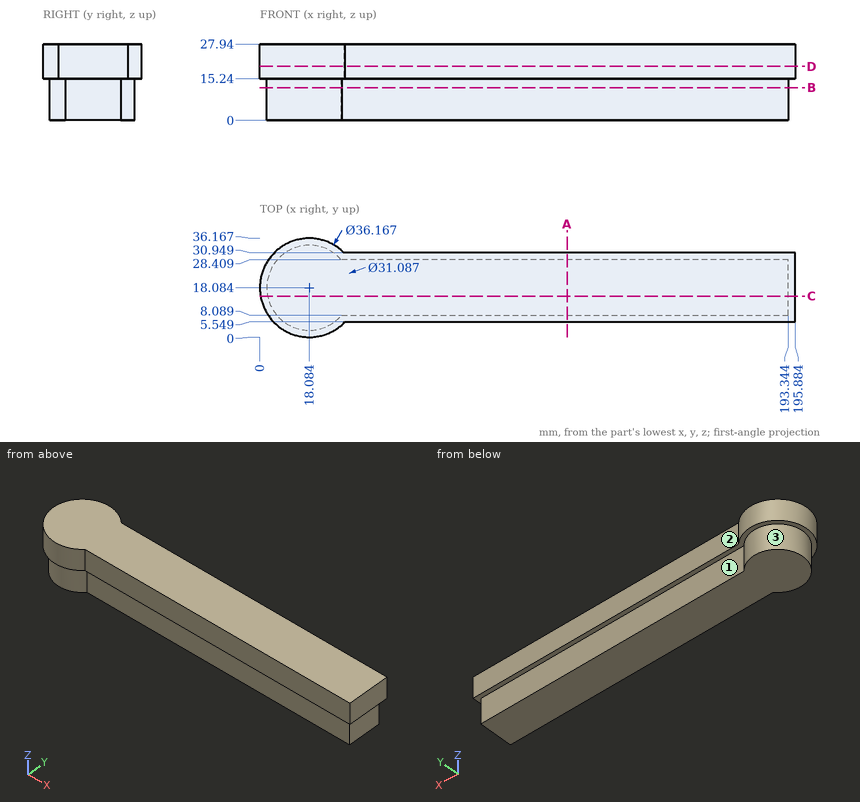
Part print with two shaded views. Sizes in mm from the minimum x, y, z corner. A direction names the side the tool comes from. Round coordinates to 2 decimals unless told otherwise and drop trailing zeros. Order: outer loops, then holes, each group sorted by start corner. A loop starts at its lowest first (then second) coordinate and runs counter-clockwise, first axis right, second up.
(1) Drill centre lines: line 1 (Y direction, x = 32, z = 22); line 2 (Y direction, x = 36.5, z = 6.25); line 3 (Z direction, x = 162, y = 30). Where is each one in solid material? Low to high.
(2) Band-saw the part on D-D (z = 19.75). List the corners of the cut face in (x, y).
(3) Band-saw the part on B-B (z = 12). List the corners of the cut face in (x, y), then the cut area to 3 significant figures.
(4) Band-saw the part on C-C (y = 15). List the corners of the cut face in (x, z) (1 decimal).
(5) Pin check, flat tips, straight feed: pin 1 (12 mm diameter, centred on x = 41, z = 9, fed in from -Y); pin 2 (8 mm diameter, centred on y = 12.5, z = 5, fed in from -X); pin 3 (7.5 mm diameter, centred on x = 81, z = 4.5, fed in from +Y). Stop position of each tip, or through.
(6) Band-saw the part on A-A (x = 112.5). List the corners of the cut face in (y, z).
(7) 3-axis set-ups, long thin cutter, end or side, ignore diameter. For the marked faces 1, 2 and 3: which of +Z, -Z, +X, -X, +Y, -Y reach the whole face in a straight line?
Verdict:
1. line 1: y = 5.55 to 30.95
1. line 2: y = 8.09 to 28.41
1. line 3: z = 15.24 to 27.94
2. outline: (30.79, 30.95) arc R18.08 ccw (long way) to (31.12, 5.55) - (195.88, 5.55) - (195.88, 30.95) - close
3. outline: (29.7, 28.41) arc R15.54 ccw (long way) to (29.99, 8.09) - (193.34, 8.09) - (193.34, 28.41) - close
3. area: 4,030 mm2
4. outline: (0.3, 15.2) - (2.8, 15.2) - (2.8, 0) - (193.3, 0) - (193.3, 15.2) - (195.9, 15.2) - (195.9, 27.9) - (0.3, 27.9) - close
5. pin 1: stops at y = 8.09
5. pin 2: stops at x = 2.62
5. pin 3: stops at y = 28.41
6. outline: (5.55, 15.24) - (8.09, 15.24) - (8.09, 0) - (28.41, 0) - (28.41, 15.24) - (30.95, 15.24) - (30.95, 27.94) - (5.55, 27.94) - close
7. face 1: -Z, +X, +Y
7. face 2: +Z, -Z, +X, +Y
7. face 3: -Z
